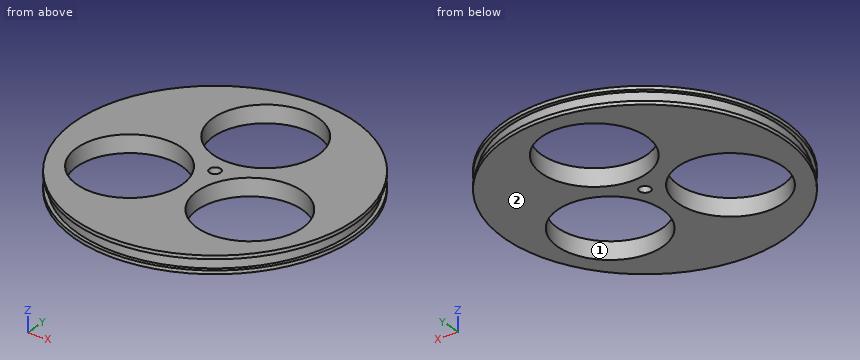
from build123d import *

# Parameters (mm, degrees)
F0_R     = 40
F0_R_2   = 1.6
F1_DEPTH = 5
F2_W     = 1
F2_H     = 3
F4_R     = 15
F5_DEPTH = 25


with BuildPart() as f1:
    # F0 (on Top) → F1 (new body)
    with BuildSketch(Plane.XY):
        Circle(F0_R)
        Circle(F0_R_2, mode=Mode.SUBTRACT)
    extrude(amount=F1_DEPTH)

    # F2 (on Right) → F3 (revolve, cut)
    with BuildSketch(Plane.YZ):
        with Locations((39.5, 2.5)):
            Rectangle(F2_W, F2_H)
    revolve(axis=Axis((0, 0, 5), (0, 0, 1)), mode=Mode.SUBTRACT)

    # F4 (on face) → F5 (cut)
    with BuildSketch(Plane.XY.offset(5)):
        with Locations((0, 20)):
            Circle(F4_R)
        with Locations((-17.320508, -10)):
            Circle(F4_R)
        with Locations((17.320508, -10)):
            Circle(F4_R)
    extrude(amount=-F5_DEPTH, mode=Mode.SUBTRACT)


solid = f1.part
For this review, take the finished solid that the model builds, in its own axes (mm). Face numbers are marked on the shaded views. Coordinates: 2 decimals unless noted, no trailing zeros. Loops run counter-clockwise (first coordinate to the right, second up) from the corner with the lowest first, then second, coordinate; pieces in that order, holes last. Notation, with made-up numbers: (42.5, 71) - (83.5, 71) arc R13 cw to (83.5, 82) - close; hole circle Ø3 at (22.25, -38). An arc over 180 degrees is marked (long way). Use a Markdown table: item, result. Add a question column.
Item 1: Mouldability with a two-part tool opening along X and no side actions: class the marked faces 1 and 2 as pulls with the +X half, pulls with the -X half, needs draft (parallel to the pull), parting line crosses it, or undercut.
Item 2: We need section C-C (z = 2.15). Give the boundary of the cut face in (x, y), and give its area (3 significant figures).
Item 3: Insertion check: pin 1 Ø6 at (x, y) = (24, -23) entering from +Z; pin 2 Ø1.5 at (x, z) = (12.5, 2.5) entering from -Y. Each pin has a flat end and moves straight along its axis. Give the tip position at first contact, or say it passes through.
Item 4: We need section A-A (x = 0). Give the boundary of the cut face in (y, z), and give its area (3 significant figures).
Item 5: We need section D-D (y = -18.5). Give the boundary of the cut face in (x, z), and give its area (3 significant figures).
Item 6: We need section B-B (y = 32). Give the boundary of the cut face in (x, z).
Item 7: For line 1 (Y direction, x = 0, z = 1.5); line 2 (Y direction, x = 5, z = 2.85); line 3 (Z direction, x = -36.5, y = -15.5), list the stretches that pass through material, from the lowest coordinate up.
Results list:
| question | item | result |
|---|---|---|
| 1 | face 1 | undercut |
| 1 | face 2 | needs draft |
| 2 | outline | circle Ø78 at (0, 0); hole circle Ø30 at (-17.32, -10); hole circle Ø30 at (0, 20); hole circle Ø3.2 at (0, 0); hole circle Ø30 at (17.32, -10) |
| 2 | area | 2,650 mm^2 |
| 3 | pin 1 | stops at z = 5 |
| 3 | pin 2 | stops at y = -37.19 |
| 4 | outline | (-40, 0) - (-1.6, 0) - (-1.6, 5) - (-40, 5) - (-40, 4) - (-39, 4) - (-39, 1) - (-40, 1) - close; (1.6, 0) - (5, 0) - (5, 5) - (1.6, 5) - close; (35, 0) - (40, 0) - (40, 1) - (39, 1) - (39, 4) - (40, 4) - (40, 5) - (35, 5) - close |
| 4 | area | 228 mm^2 |
| 5 | outline | (-35.46, 0) - (-29.68, 0) - (-29.68, 5) - (-35.46, 5) - (-35.46, 4) - (-34.33, 4) - (-34.33, 1) - (-35.46, 1) - close; (-4.96, 0) - (4.96, 0) - (4.96, 5) - (-4.96, 5) - close; (29.68, 0) - (35.46, 0) - (35.46, 1) - (34.33, 1) - (34.33, 4) - (35.46, 4) - (35.46, 5) - (29.68, 5) - close |
| 5 | area | 101 mm^2 |
| 6 | outline | (-24, 0) - (-9, 0) - (-9, 5) - (-24, 5) - (-24, 4) - (-22.29, 4) - (-22.29, 1) - (-24, 1) - close; (9, 0) - (24, 0) - (24, 1) - (22.29, 1) - (22.29, 4) - (24, 4) - (24, 5) - (9, 5) - close |
| 7 | line 1 | y = -39 to -1.6, 1.6 to 5, 35 to 39 |
| 7 | line 2 | y = -38.68 to -18.56, -1.44 to 5.86, 34.14 to 38.68 |
| 7 | line 3 | z = 0 to 1, 4 to 5 |
